Design review of the part built by this model. Coordinates are the model's own, in mm. A direction names the side the tool comes from. Coordinates: 2 decimals unless noted, no trailing zeros. Order: outer loops, then holes, each group sorted by start corner. A loop starts at its lowest first (then second) coordinate and runs counter-clockwise, first axis right, second up. Notation, with made-up numbers: M -22,-37.75 L 31,-37.75 A10 ccw 31,-31.75 Z; hole C -33,-11 d11. An arc over 180 degrees is marked long. Answer as a JSON object with one key per item and string values.
from build123d import *

# Parameters (mm, degrees)
F0_W     = 76.2
F0_H     = 38.1
F1_DEPTH = 63.5
F2_R     = 12.7
F3_T     = -1.524
F4_W     = 2.286
F4_H     = 40.64
F5_DEPTH = 1.524
F6_R     = 1.14299


# Not quite as in the source:
# - a fillet or chamfer is up to 0.001 mm smaller than in the source, because OpenCascade refuses the exact size


with BuildPart() as f1:
    # F0 (on Top) → F1 (new body)
    with BuildSketch(Plane.XY):
        Rectangle(F0_W, F0_H)
    extrude(amount=F1_DEPTH)

    # F2
    f2_edges = [f1.edges().sort_by_distance(p)[0] for p in [
        (38.1, -19.05, 31.75),
        (38.1, 19.05, 31.75),
        (-38.1, -19.05, 31.75),
        (-38.1, 19.05, 31.75),
    ]]
    fillet(f2_edges, radius=F2_R)

    # F3
    f3_openings = [f1.faces().sort_by_distance(p)[0] for p in [
        (0, 0, 63.5),
    ]]
    offset(amount=F3_T, openings=f3_openings)

    # F4 (on face) → F5 (cut, through all)
    with BuildSketch(Plane(origin=(0, 19.05, 0), x_dir=(-1, 0, 0), z_dir=(0, 1, 0))):
        with Locations((0, 31.75)):
            Rectangle(F4_W, F4_H)
    extrude(amount=-F5_DEPTH, mode=Mode.SUBTRACT)

    # F6 (radius 1.143 in the source; OpenCascade refuses exactly that, so slightly less here)
    f6_edges = [f1.edges().sort_by_distance(p)[0] for p in [
        (1.143, 18.288, 52.07),
        (-1.143, 18.288, 52.07),
        (1.143, 18.288, 11.43),
        (-1.143, 18.288, 11.43),
    ]]
    fillet(f6_edges, radius=F6_R)


solid = f1.part
1) Add section D-D (z = 14.5). State the section outline as (x, y) points, and give its area (3 significant figures).
Taken from the geometry:
{"outline": "M -38.1,-6.35 A12.7 ccw -25.4,-19.05 L 25.4,-19.05 A12.7 ccw 38.1,-6.35 L 38.1,6.35 A12.7 ccw 25.4,19.05 L 1.14,19.05 L 1.14,17.53 L 25.4,17.53 A11.18 cw 36.58,6.35 L 36.58,-6.35 A11.18 cw 25.4,-17.53 L -25.4,-17.53 A11.18 cw -36.58,-6.35 L -36.58,6.35 A11.18 cw -25.4,17.53 L -1.14,17.53 L -1.14,19.05 L -25.4,19.05 A12.7 ccw -38.1,6.35 Z", "area": "304 mm2"}
2) Insertion check: pin 1 Ø6 at (y, z) = (-15, 31.5) entering from -X; pin 2 Ø1.2 at (y, z) = (18, 27) entering from -X; pin 3 Ø17.5 at (x, y) = (13.5, -1.5) entering from +Z. Each pin has a flat end and moves straight along its axis. Give the tip position at first contact, or say it passes through.
Taken from the geometry:
{"pin 1": "stops at x = -36.77", "pin 2": "stops at x = -31.66", "pin 3": "stops at z = 1.52"}
3) Add section B-B (x = -21). State the section outline as (y, z) points, and give its area (3 significant figures).
Taken from the geometry:
{"outline": "M -19.05,0 L 19.05,0 L 19.05,63.5 L 17.53,63.5 L 17.53,1.52 L -17.53,1.52 L -17.53,63.5 L -19.05,63.5 Z", "area": "247 mm2"}
4) Mouldability with a two-part tool opening along X and no side actions: class faces 3 (the flat face through (-38.1, 0, 31)), 4 (the flat face through (-1, 0, 0)), 5 (the cylindrical face through (33.215, -14.339, 32.946)) as released by +X, released by -X, zero draft, split by the parting line, or undercut.
Taken from the geometry:
{"face 3": "released by -X", "face 4": "zero draft", "face 5": "undercut"}
5) To check wall thickness, follow L1, parallel to Y at x = -20.5, z = 24; L2, parallel to X at y = 7, z = 22. State the ranges of each line that lie inside material, in increasing order.
Taken from the geometry:
{"L1": "y = -19.05 to -17.53, 17.53 to 19.05", "L2": "x = -38.08 to -36.56, 36.56 to 38.08"}
6) Add section C-C (y = 2.5). State the section outline as (x, z) points.
Taken from the geometry:
{"outline": "M -38.1,0 L 38.1,0 L 38.1,63.5 L 36.58,63.5 L 36.58,1.52 L -36.58,1.52 L -36.58,63.5 L -38.1,63.5 Z"}
7) Tool access review of faces 1 (the flat face through (36.576, 0, 32)), 2 (the cylindrical face through (34.48, 15.23, 32.19)): name each direction out of +Z, -Z, +X, -X, +Y, -Y from which nothing blocks a thin tool from reaching the whole face with its end or side.
Taken from the geometry:
{"face 1": "+Z", "face 2": "+Z, -Z, +X, +Y"}
8) Add section A-A (z = 59.5). State the section outline as (x, y) points, and give its area (3 significant figures).
Taken from the geometry:
{"outline": "M -38.1,-6.35 A12.7 ccw -25.4,-19.05 L 25.4,-19.05 A12.7 ccw 38.1,-6.35 L 38.1,6.35 A12.7 ccw 25.4,19.05 L -25.4,19.05 A12.7 ccw -38.1,6.35 Z; hole M -36.58,-6.35 A11.18 ccw -25.4,-17.53 L 25.4,-17.53 A11.18 ccw 36.58,-6.35 L 36.58,6.35 A11.18 ccw 25.4,17.53 L -25.4,17.53 A11.18 ccw -36.58,6.35 Z", "area": "308 mm2"}
